Verification items for the finished model (mm, model axes). Face numbers are marked on the shaded views. Round coordinates to 2 decimals unless told otherwise and drop trailing zeros. Write each loop counter-clockwise with the first axis right and the second up, starting at its lowest first coordinate (ties: lowest second). Pieces come first, ordered by that corner, then holes. Notation, with made-up numbers: M -12,32.25 L 47,32.25 A17 ccw 47,56.25 Z; hole C 63.25,42.25 d5. An arc over 180 degrees is marked long. One line per item, written item: value. Start each with the question number.
Item 1: Gauge pin test, flat ends, axial feed: pin 1 (2 mm diameter, centred on x = -2, y = 9, fed in from +Z); pin 2 (2 mm diameter, centred on x = -1.5, y = 22, fed in from +Z); pin 3 (3 mm diameter, centred on x = 0, z = 6.5, fed in from -Y). Record the tip position at first contact, or that the pin passes through.
Item 2: Section check D-D, the plane x = -2.5. Record the cut outline in (y, z) (3 decimals), then the cut area to 3 significant figures.
Item 3: Draft check along Z on the marked faces 1, 2 and 3. Enter one of: +Z half, -Z half, draft (parallel to the pull), parting line (faces both ways), or undercut.
Item 4: Section check B-B, the plane z = 5.75. Record the cut outline in (x, y).
Item 5: Section check C-C, the plane y = 10.5. Record the cut outline in (x, z), then the cut area to 3 significant figures.
Item 6: Thickness scan on probe 1 along Z at (x, y) = (0, 24.5); probe 2 along X at (y, z) = (0.55, 6.5); probe 3 along Y at (x, z) = (2.5, 4). Record the ranges inside material, lowest first. Write a range as from..to.
Item 7: Section check A-A, the plane x = 0. Record the cut outline in (y, z) (3 decimals).
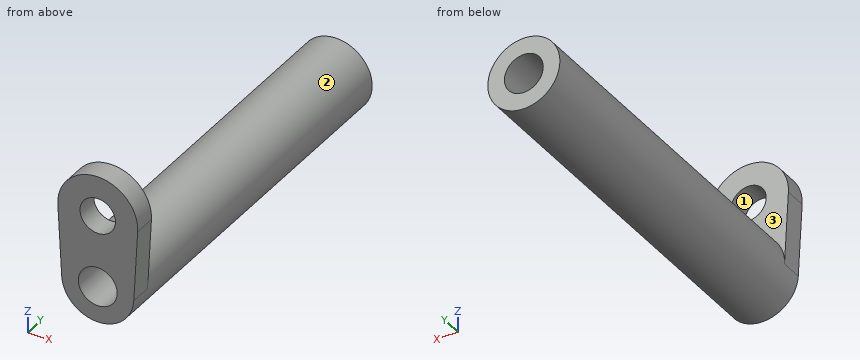
from build123d import *

# Parameters (mm, degrees)
SKETCH1_R           = 3.25
SKETCH1_R_2         = 1.75
BOSS_EXTRUDE1_DEPTH = 34.625
SKETCH2_R           = 1.75
SKETCH2_R_2         = 1.6
BOSS_EXTRUDE2_DEPTH = 2


with BuildPart() as part:
    # Sketch1 → Boss-Extrude1 (new body)
    with BuildSketch(Plane(origin=(0, 0, 0), x_dir=(1, 0, 0), z_dir=(0, 1, 0))):
        with Locations(Location((0, 0, 0), (0, 0, 180))):
            Circle(SKETCH1_R)
        with Locations(Location((0, 0, 0), (0, 0, 180))):
            Circle(SKETCH1_R_2, mode=Mode.SUBTRACT)
    extrude(amount=BOSS_EXTRUDE1_DEPTH)

    # Sketch2 → Boss-Extrude2 (add)
    with BuildSketch(Plane(origin=(0, 0, 0), x_dir=(1, 0, 0), z_dir=(0, 1, 0))):
        with BuildLine():
            Line((-3.594777277, -6.306153846), (-3.245285041, 0.175))
            ThreePointArc((-3.245285041, 0.175), (0, 3.25), (3.245285041, 0.175))
            Line((3.245285041, 0.175), (3.594777277, -6.306153846))
            ThreePointArc((3.594777277, -6.306153846), (0, -10.1), (-3.594777277, -6.306153846))
        make_face()
        with Locations(Location((0, 0, 0), (0, 0, 180))):
            Circle(SKETCH2_R, mode=Mode.SUBTRACT)
        with Locations(Location((0, -6.5, 0), (0, 0, 270))):
            Circle(SKETCH2_R_2, mode=Mode.SUBTRACT)
    extrude(amount=BOSS_EXTRUDE2_DEPTH)


solid = part.part
Response values:
1. pin 1: stops at z = 3.09
1. pin 2: stops at z = 3.21
1. pin 3: passes through
2. outline: M 0,-2.077 L 34.625,-2.077 L 34.625,2.077 L 2,2.077 L 2,9.09 L 0,9.09 Z
2. area: 158 mm2
3. face 1: undercut
3. face 2: parting line
3. face 3: draft
4. outline: M -3.56,0 L -1.41,0 L -1.41,2 L -3.56,2 Z; M 1.41,0 L 3.56,0 L 3.56,2 L 1.41,2 Z
5. outline: C 0,0 d6.5; hole C 0,0 d3.5
5. area: 23.6 mm2
6. probe 1: z = -3.25..-1.75, 1.75..3.25
6. probe 2: x = -3.6..-1.6, 1.6..3.6
6. probe 3: y = 0..2
7. outline: M 0,-3.25 L 34.625,-3.25 L 34.625,-1.75 L 0,-1.75 Z; M 0,1.75 L 34.625,1.75 L 34.625,3.25 L 2,3.25 L 2,4.9 L 0,4.9 Z; M 0,8.1 L 2,8.1 L 2,10.1 L 0,10.1 Z
